Geometry check sheet. Reference: the model listing, model coordinates, mm. A direction names the side the tool comes from. Give positions to 0.01 mm unless a question says otherwise; leave off trailing zeros. Order: outer loops, then holes, each group sorted by start corner. A loop starts at its lowest first (then second) coordinate and runs counter-clockwise, first axis right, second up. Notation, with made-up numbers: M -28.75,86 L -16.75,86 A21 ccw -16.75,91 Z; hole C 35,54 d5. An arc over 180 degrees is marked long. Use CSV: the item, a comma, the result in double quotes. Start each with the question number.
from build123d import *

# Parameters (mm, degrees)
SKETCH_1_R          = 11.38
EXTRUDE_1_DEPTH     = 7.09
SKETCH_2_R          = 10
CUT_EXTRUDE_1_DEPTH = 5.09
SKETCH_3_R          = 3.46
EXTRUDE_2_DEPTH     = 6.1
SKETCH_4_R          = 3.46
EXTRUDE_3_DEPTH     = 5.18
EXTRUDE_3_DRAFT     = 56
SKETCH_5_R          = 8.873129811
CUT_EXTRUDE_2_DEPTH = 5.18
CUT_EXTRUDE_2_DRAFT = -51
SKETCH_6_R          = 2.476362541
CUT_EXTRUDE_3_DEPTH = 3.92


with BuildPart() as part:
    # 草图1 → 凸台-拉伸1 (new body)
    with BuildSketch(Plane(origin=(0, 0, 0), x_dir=(1, 0, 0), z_dir=(0, 1, 0))):
        with Locations(Location((0, 0, 0), (0, 0, 270))):  # turned: the seam where the file's is
            Circle(SKETCH_1_R)
    extrude(amount=EXTRUDE_1_DEPTH)

    # 草图2 → 切除-拉伸1 (cut)
    with BuildSketch(Plane(origin=(0, 7.09, 0), x_dir=(1, 0, 0), z_dir=(0, 1, 0))):
        with Locations(Location((0, 0, 0), (0, 0, 270))):  # turned: the seam where the file's is
            Circle(SKETCH_2_R)
    extrude(amount=-CUT_EXTRUDE_1_DEPTH, mode=Mode.SUBTRACT)

    # 草图3 → 凸台-拉伸2 (add)
    with BuildSketch(Plane(origin=(0, 2, 0), x_dir=(1, 0, 0), z_dir=(0, 1, 0))):
        with Locations(Location((0, 0, 0), (0, 0, 270))):  # turned: the seam where the file's is
            Circle(SKETCH_3_R)
    extrude(amount=EXTRUDE_2_DEPTH)


with BuildPart() as extrude_3_tool:
    # 草图4 → 凸台-拉伸3 (with draft: the straight prism first)
    with BuildSketch(Plane(origin=(0, 6.27, 0), x_dir=(1, 0, 0), z_dir=(0, 1, 0))):
        with Locations(Location((0, 0, 0), (0, 0, 270))):  # turned: the seam where the file's is
            Circle(SKETCH_4_R)
    extrude(amount=-EXTRUDE_3_DEPTH)
    # 凸台-拉伸3: the draft: its side faces are tilted about the plane it starts from
    extrude_3_sides = [extrude_3_tool.faces().sort_by_distance(p)[0] for p in [
        (0, 3.68, -3.46),
    ]]
    draft(extrude_3_sides, Plane(origin=(0, 6.27, 0), x_dir=(1, 0, 0), z_dir=(0, 1, 0)), EXTRUDE_3_DRAFT)


with BuildPart() as part_1:
    add(part.part)

    # 凸台-拉伸3: add extrude_3_tool
    add(extrude_3_tool.part)


with BuildPart() as cut_extrude_2_tool:
    # 草图5 → 切除-拉伸2 (with draft: the straight prism first)
    with BuildSketch(Plane.XZ):
        Circle(SKETCH_5_R)
    extrude(amount=-CUT_EXTRUDE_2_DEPTH)
    # 切除-拉伸2: the draft: its side faces are tilted about the plane it starts from
    cut_extrude_2_sides = [cut_extrude_2_tool.faces().sort_by_distance(p)[0] for p in [
        (-8.873129811, 2.59, 0),
    ]]
    draft(cut_extrude_2_sides, Plane.XZ, CUT_EXTRUDE_2_DRAFT)


with BuildPart() as part_2:
    add(part_1.part)

    # 切除-拉伸2: cut by cut_extrude_2_tool
    add(cut_extrude_2_tool.part, mode=Mode.SUBTRACT)

    # 草图6 → 切除-拉伸3 (cut, through all)
    with BuildSketch(Plane.XZ.offset(-5.18)):
        with Locations(Location((0, 0, 0), (0, 0, 270))):  # turned: the seam where the file's is
            Circle(SKETCH_6_R)
    extrude(amount=-CUT_EXTRUDE_3_DEPTH, mode=Mode.SUBTRACT)


solid = part_2.part
(1) Go/stop test with flat-tipped pins: P1, Ø10, axis at x = 0.5, z = -2, coming from the +Y side; P2, Ø1.5, axis at y = 6.5, z = 8.5, coming from the +X side; P3, Ø1.5, axis at x = -5.5, y = 3, coming from the +Z side; P4, Ø5.5, axis at x = 0, z = 0, coming from the -Y side. Record where each tip stops, or that it passes through.
(2) Draft check along X on faces 3 (the face through (-9.76, 4.58, -2.17)), 4 (the face through (-10.096, 3.495, 5.251)), 5 (the face through (-8, 7.09, 7)). Enter one of: +X half, -X half, draft (parallel to the pull), parting line (faces both ways), or undercut.
(3) Sectioned sample at B-B on z = 0. Record the cut outline in (x, y), then the cut area to 3 significant figures.
(4) Sectioned sample at C-C on y = 5.5. Record the cut outline in (x, z).
(5) Sectioned sample at A-A on x = 0. Record the cut outline in (y, z), then the cut area to 3 significant figures.
(6) Thickness scan on line 1 (Z direction, x = 3.25, y = 3.25); line 2 (X direction, y = 4.75, z = 0.25); line 3 (X direction, y = 6.95, z = 0). Record the ranges inside material, lowest first.
(7) Access from +Z, -Z, +X, -X, +Y, -Y to the whole of each face (thin tool, end or side, straight path). Record for faces 1 (the face through (-1.325, 7.172, 3.196)), 2 (the face through (-2.3, 8.1, 1.5)).
(8) Sectioned sample at D-D on y = 4. Record the cut outline in (x, z), then the cut area to 3 significant figures.
Responses:
1,P1,"y = 8.1"
1,P2,"x = 8.33"
1,P3,"z = 10.34"
1,P4,"y = 4.96"
2,face 3,"undercut"
2,face 4,"parting line"
2,face 5,"draft"
3,outline,"M -11.38,0 L -8.87,0 L -2.48,5.18 L -2.48,8.1 L -3.46,8.1 L -3.46,6.27 L -9.79,2 L -10,2 L -10,7.09 L -11.38,7.09 Z; M 2.48,5.18 L 8.87,0 L 11.38,0 L 11.38,7.09 L 10,7.09 L 10,2 L 9.79,2 L 3.46,6.27 L 3.46,8.1 L 2.48,8.1 Z"
3,area,"55.6 mm2"
4,outline,"C 0,0 d22.76; C 0,0 d9.2; hole C 0,0 d20; hole C 0,0 d4.95"
5,outline,"M 0,-11.38 L 7.09,-11.38 L 7.09,-10 L 2,-10 L 2,-9.79 L 6.27,-3.46 L 8.1,-3.46 L 8.1,-2.48 L 5.18,-2.48 L 0,-8.87 Z; M 0,8.87 L 5.18,2.48 L 8.1,2.48 L 8.1,3.46 L 6.27,3.46 L 2,9.79 L 2,10 L 7.09,10 L 7.09,11.38 L 0,11.38 Z"
5,area,"55.6 mm2"
6,line 1,"-10.91 to -9.46, -7.24 to -3.61, 3.61 to 7.24, 9.46 to 10.91"
6,line 2,"-11.38 to -10, -5.71 to -3, 3 to 5.71, 10 to 11.38"
6,line 3,"-11.38 to -10, -3.46 to -2.48, 2.48 to 3.46, 10 to 11.38"
7,face 1,"+Y"
7,face 2,"+Z, -Z, +X, -X, +Y"
8,outline,"C 0,0 d22.76; C 0,0 d13.65; hole C 0,0 d20; hole C 0,0 d7.87"
8,area,"190 mm2"
